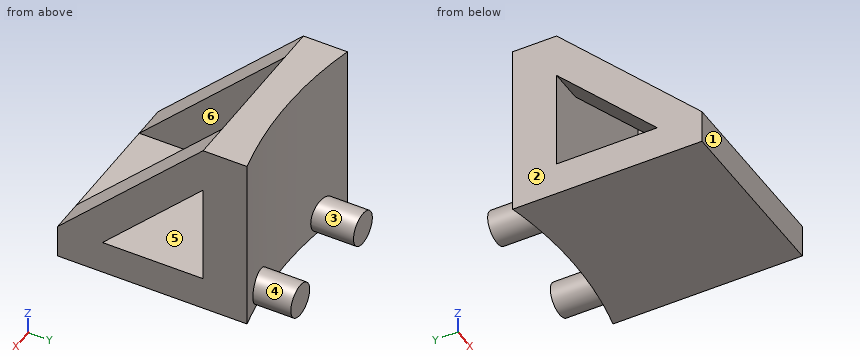
from build123d import *

# Parameters (mm, degrees)
F1_DEPTH      = 50.8
F3_DEPTH      = 15.875
F3_DEPTH_BACK = 15.875
F4_DEPTH      = 25.4
F4_DEPTH_BACK = 25.4
F5_R          = 4.7625
F6_DEPTH      = 12.7


with BuildPart() as f1:
    # F0 (on Top) → F1 (new body)
    with BuildSketch(Plane.XY):
        with BuildLine():
            Line((-25.4, -50.8), (25.4, -50.8))
            Line((25.4, -50.8), (25.4, 2.9417960125))
            ThreePointArc((25.4, 2.9417960125), (0, 0), (-25.4, 2.9417960125))
            Line((-25.4, 2.9417960125), (-25.4, -50.8))
        make_face()
    extrude(amount=F1_DEPTH)

    # F2 (on Right) → F3 (cut, two sides)
    with BuildSketch(Plane.YZ) as f3_sk:
        Polygon((-9.525, 50.8), (-50.8, 9.525), (-38.1, 9.525), (-9.525, 38.1), align=None)
        Polygon((-9.525, 38.1), (-38.1, 9.525), (-9.525, 9.525), align=None)
        Polygon((-50.8, 50.8), (-50.8, 9.525), (-9.525, 50.8), align=None)
    extrude(amount=F3_DEPTH, mode=Mode.SUBTRACT)
    extrude(f3_sk.sketch, amount=-F3_DEPTH_BACK, mode=Mode.SUBTRACT)

    # F2 (on Right) → F4 (cut, two sides)
    with BuildSketch(Plane.YZ) as f4_sk:
        Polygon((-9.525, 38.1), (-38.1, 9.525), (-9.525, 9.525), align=None)
        Polygon((-50.8, 50.8), (-50.8, 9.525), (-9.525, 50.8), align=None)
    extrude(amount=-F4_DEPTH, mode=Mode.SUBTRACT)
    extrude(f4_sk.sketch, amount=F4_DEPTH_BACK, mode=Mode.SUBTRACT)

    # F5 (on Front) → F6 (join)
    with BuildSketch(Plane.XZ):
        with Locations((-15.875, 4.7625)):
            Circle(F5_R)
        with Locations((15.875, 4.7625)):
            Circle(F5_R)
    extrude(amount=-F6_DEPTH)


solid = f1.part
Source: CAD feature listing. Evaluate the final solid. Frame: model axes, mm. Face numbers are marked on the shaded views. A direction names the side the tool comes from. Round coordinates to 2 decimals unless told otherwise and drop trailing zeros. Order: outer loops, then holes, each group sorted by start corner. A loop starts at its lowest first (then second) coordinate and runs counter-clockwise, first axis right, second up. Notation, with made-up numbers: (54, 34.25) - (94, 34.25) arc R18 ccw to (94, 61.25) - close; hole circle Ø4 at (-16.75, 55.5). An arc over 180 degrees is marked (long way). Use a Markdown table: item, result. Add a question column.
1. Section query C-C (y = -27). Return the cut outline in (x, z) (3 decimals).
2. Section query B-B (x = -22). Return the cut outline in (y, z) (1 decimal).
3. Mould query, pull axis X, two halves, no side actions, for the marked faces 1, 2 and 3. Classes: +X half, -X half, draft (parallel to the pull), parting line (faces both ways), or undercut.
4. First-contact query: pin 1 (8 mm diameter, centred on x = 7, y = -18, fed in from +Z) (3 decimals); pin 2 (5 mm diameter, centred on x = 6, z = 39.5, fed in from +Y); pin 3 (1 mm diameter, centred on x = -10.5, z = 29, fed in from +Y). Flat tips, straight axial feed; report the tip coordinate or a pass-through.
5. Set-up query: the marked faces 4, 5 and 6. Return all of +Z, -Z, +X, -X, +Y, -Y with unobstructed straight access to the full face (end or side cutting, diameter ignored); none if empty.
6. Section query D-D (x = -13.5). Return the cut outline in (y, z) (3 decimals), then the cut area to 3 significant figures.
7. Section query A-A (z = 24.5). Return the cut outline in (x, y) (3 decimals).
8. Line query: probe 1 along X at (y, z) = (-13, 47) (3 decimals); probe 2 along Z at (x, y) = (16.5, -36.5) (3 decimals); probe 3 along Z at (x, y) = (-11.5, -17) (3 decimals). Output: solid intervals per line, ascending.
Derived:
| question | item | result |
|---|---|---|
| 1 | outline | (-25.4, 0) - (25.4, 0) - (25.4, 9.525) - (-25.4, 9.525) - close; (-25.4, 20.625) - (-15.875, 20.625) - (-15.875, 33.325) - (-25.4, 33.325) - close; (15.875, 20.625) - (25.4, 20.625) - (25.4, 33.325) - (15.875, 33.325) - close |
| 2 | outline | (-50.8, 0) - (2.2, 0) - (2.2, 50.8) - (-9.5, 50.8) - (-50.8, 9.5) - close; hole (-38.1, 9.5) - (-9.5, 9.5) - (-9.5, 38.1) - close |
| 3 | face 1 | draft |
| 3 | face 2 | -X half |
| 3 | face 3 | undercut |
| 4 | pin 1 | z = 9.525 |
| 4 | pin 2 | y = 0.33 |
| 4 | pin 3 | y = 0.55 |
| 5 | face 4 | +Y |
| 5 | face 5 | none |
| 5 | face 6 | +Z, -Y |
| 6 | outline | (-50.8, 0) - (0.823, 0) - (0.823, 0.634) - (12.7, 0.634) - (12.7, 8.891) - (0.823, 8.891) - (0.823, 50.8) - (-9.525, 50.8) - (-9.525, 9.525) - (-50.8, 9.525) - close |
| 6 | area | 1,020 mm2 |
| 7 | outline | (-25.4, -35.825) - (-15.875, -35.825) - (-15.875, -23.125) - (-25.4, -23.125) - close; (-25.4, -9.525) - (25.4, -9.525) - (25.4, 2.942) arc R111.125 cw to (-25.4, 2.942) - close; (15.875, -35.825) - (25.4, -35.825) - (25.4, -23.125) - (15.875, -23.125) - close |
| 8 | probe 1 | -25.4 to -15.875, 15.875 to 25.4 |
| 8 | probe 2 | 0 to 9.525, 11.125 to 23.825 |
| 8 | probe 3 | 0 to 9.525 |
